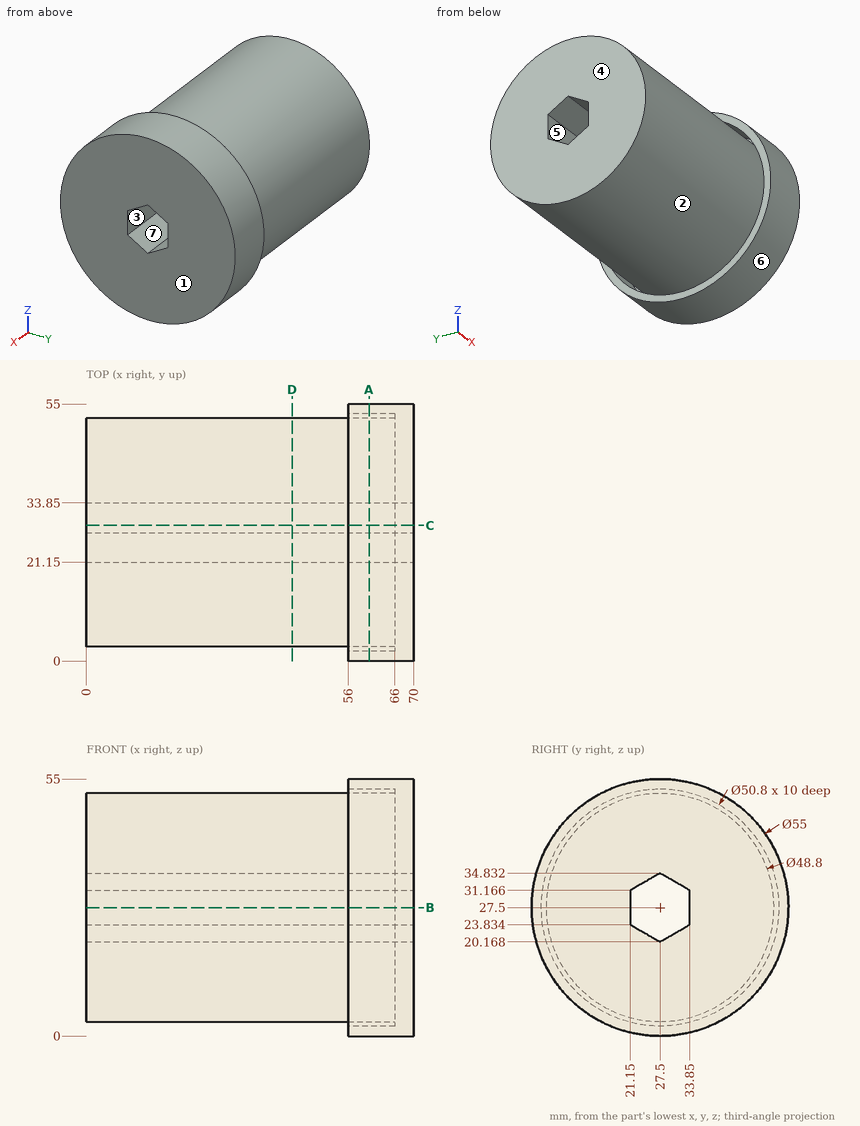
For this review, use the dimensioned drawing (mm, ordinates from the lowest corner) and the shaded views. A direction names the side the tool comes from. Coordinates: 2 decimals unless noted, no trailing zeros. Loops run counter-clockwise (first coordinate to the right, second up) from the corner with the lowest first, then second, coordinate; pieces in that order, holes last. Notation, with made-up numbers: (-40, -0.75) -> (-2, -0.75) arc R25 cw to (-2, 13.25) -> close; hole circle Ø8 at (-30, -16.75). An arc over 180 degrees is marked (long way). Use a Markdown table: item, result. Add a question column.
Item 1: We need section C-C, the plane y = 29. Write out the cut boundary in (x, z) (1 decimal).
Item 2: Wall thickness on L1, parallel to Y at x = 61.25, z = 27.5; L2, parallel to Z at x = 64, y = 38 (1 decimal); L3, parallel to Z at x = 63, y = 27 (1 decimal): over which ranges is each line inside the solid? List them lowest first. Write a range as from..to.
Item 3: The part is to be moulded in two halves that separate along Y. For the marked faces 4, 5, 6 and 7, say which applies: +Y half, -Y half, draft (parallel to the pull), parting line (faces both ways), or undercut.
Item 4: We need section A-A, the plane x = 60.5. Write out the cut boundary in (y, z), and give its area (3 significant figures).
Item 5: We need section B-B, the plane z = 27.5. Write out the cut boundary in (x, y).
Item 6: Clearance check with flat-ended pins moving along their axes: P1, Ø2, axis at x = 49.5, y = 10, coming from the +Z side (1 decimal); P2, Ø1, axis at x = 56, y = 29.5, coming from the +Z side; P3, Ø5, axis at x = 47, z = 48, coming from the -Y side; P4, Ø16.5, axis at y = 18.5, z = 30, coming from the -X side. State where each tip first meets the part, or that it passes through.
Item 7: We need section D-D, the plane x = 44. Write out the cut boundary in (y, z), and give its area (3 significant figures).
Item 8: Machinability: for the marked faces 1, 2 and 3, which of the approach directions +Z, -Z, +X, -X, +Y, -Y give a long, thin tool a straight path to every point of the face, cutting with its end or side? Answer none if there is none.
Numbers:
| question | item | result |
|---|---|---|
| 1 | outline | (0, 3.1) -> (66, 3.1) -> (66, 2.1) -> (56, 2.1) -> (56, 0) -> (70, 0) -> (70, 21) -> (0, 21) -> close; (0, 34) -> (70, 34) -> (70, 55) -> (56, 55) -> (56, 52.9) -> (66, 52.9) -> (66, 51.9) -> (0, 51.9) -> close |
| 2 | L1 | y = 0..2.1, 3.1..21.15, 33.85..51.9, 52.9..55 |
| 2 | L2 | z = 2.1..4.4, 5.5..49.5, 50.6..52.9 |
| 2 | L3 | z = 0..2.1, 3.1..20.5, 34.5..51.9, 52.9..55 |
| 3 | face 4 | draft |
| 3 | face 5 | undercut |
| 3 | face 6 | parting line |
| 3 | face 7 | undercut |
| 4 | outline | circle Ø55 at (27.5, 27.5); circle Ø48.8 at (27.5, 27.5); hole circle Ø50.8 at (27.5, 27.5); hole (21.15, 23.83) -> (27.5, 20.17) -> (33.85, 23.83) -> (33.85, 31.17) -> (27.5, 34.83) -> (21.15, 31.17) -> close |
| 4 | area | 2,080 mm^2 |
| 5 | outline | (0, 3.1) -> (66, 3.1) -> (66, 2.1) -> (56, 2.1) -> (56, 0) -> (70, 0) -> (70, 21.15) -> (0, 21.15) -> close; (0, 33.85) -> (70, 33.85) -> (70, 55) -> (56, 55) -> (56, 52.9) -> (66, 52.9) -> (66, 51.9) -> (0, 51.9) -> close |
| 6 | P1 | stops at z = 45.5 |
| 6 | P2 | stops at z = 54.96 |
| 6 | P3 | stops at y = 11.03 |
| 6 | P4 | stops at x = 0 |
| 7 | outline | circle Ø48.8 at (27.5, 27.5); hole (21.15, 23.83) -> (27.5, 20.17) -> (33.85, 23.83) -> (33.85, 31.17) -> (27.5, 34.83) -> (21.15, 31.17) -> close |
| 7 | area | 1,730 mm^2 |
| 8 | face 1 | +Z, -Z, +X, +Y, -Y |
| 8 | face 2 | -X |
| 8 | face 3 | +X, -X |
